Autodesk Fusion 360 part; units mm, degrees
sketch "Sketch1" plane through (0, 0, 0) normal (0, 1, 0) x (1, 0, 0)
  line L0 (35, 20) -> (-35, 20)
  line L1 (-40, 15) -> (-40, -15)
  line L2 (-35, -20) -> (35, -20)
  line L3 (40, -15) -> (40, 15)
  line L4 (40, 20) -> (-40, -20) construction
  line L5 (-40, 20) -> (40, -20) construction
  arc A0 (-35, 20) -> (-40, 15) centre (-35, 15) ccw
  arc A1 (40, 15) -> (35, 20) centre (35, 15) ccw
  arc A2 (35, -20) -> (40, -15) centre (35, -15) ccw
  arc A3 (-40, -15) -> (-35, -20) centre (-35, -15) ccw
  line L6 (-36, 15) -> (-36, -15)
  arc A4 (-36, -15) -> (-35, -16) centre (-35, -15) ccw
  line L7 (-35, -16) -> (35, -16)
  arc A5 (35, -16) -> (36, -15) centre (35, -15) ccw
  line L8 (36, -15) -> (36, 15)
  arc A6 (36, 15) -> (35, 16) centre (35, 15) ccw
  line L9 (35, 16) -> (-35, 16)
  arc A7 (-35, 16) -> (-36, 15) centre (-35, 15) ccw
  dimension "d1" = 80
  dimension "d2" = 40
  dimension "d3" = 5
  dimension "d4" = -4
extrude "Extrude1" add sketch "Sketch1" along normal blind 4 contours L6 A4 L7 A5 L8 A6 L9 A7
extrude "Extrude2" add sketch "Sketch1" along normal blind 20
sketch "Sketch2" plane through (0, 20, 0) normal (0, 1, 0) x (-1, 0, 0)
  arc A0 (35, -16) -> (36, -15) centre (35, -15) ccw
  line L0 (35, -16) -> (-35, -16)
  arc A1 (-36, -15) -> (-35, -16) centre (-35, -15) ccw
  line L1 (-36, -15) -> (-36, 15)
  arc A2 (-35, 16) -> (-36, 15) centre (-35, 15) ccw
  line L2 (-35, 16) -> (35, 16)
  arc A3 (36, 15) -> (35, 16) centre (35, 15) ccw
  line L3 (36, 15) -> (36, -15)
  arc A4 (40, 15) -> (35, 20) centre (35, 15) ccw
  line L4 (35, 20) -> (-35, 20)
  arc A5 (-35, 20) -> (-40, 15) centre (-35, 15) ccw
  line L5 (-40, 15) -> (-40, -15)
  arc A6 (-40, -15) -> (-35, -20) centre (-35, -15) ccw
  line L6 (-35, -20) -> (35, -20)
  arc A7 (35, -20) -> (40, -15) centre (35, -15) ccw
  line L7 (40, -15) -> (40, 15)
  line L8 (37.12, 17.12) -> (-37.12, 17.12)
  line L9 (-37.12, 17.12) -> (-37.12, -17.12)
  line L10 (-37.12, -17.12) -> (37.12, -17.12)
  line L11 (37.12, -17.12) -> (37.12, 17.12)
  line L12 (37.12, 17.12) -> (-37.12, -17.12) construction
  line L13 (-37.12, 17.12) -> (37.12, -17.12) construction
  dimension "d9" = 74.24
  dimension "d10" = 34.24
hole "Hole1" at (37.12, 20, 17.12) at (-37.12, 20, 17.12) at (-37.12, 20, -17.12) at (37.12, 20, -17.12) direction (0, -1, 0) diameter 1.471 depth 11 tip angle 118
Verification items for the finished model (mm, model axes). A direction names the side the tool comes from. Round coordinates to 2 decimals unless told otherwise and drop trailing zeros. Loops run counter-clockwise (first coordinate to the right, second up) from the corner with the lowest first, then second, coordinate; pieces in that order, holes last. Notation, with made-up numbers: (12, 47) - (44, 47) arc R26 ccw to (44, 62) - close; hole circle Ø6 at (6.25, 38). An arc over 180 degrees is marked (long way). Write item = value, one per line.
Q1. Tool access check on faces 5 (the flat face through (0, 10, 20)), 6 (the cylindrical face through (36.9, 14.42, -16.42)). Record the directions out of +Z, -Z, +X, -X, +Y, -Y that give a thin tool (end or side, any length) a straight path to the whole face; none if there is none.
Here are the results:
face_5 = +Z, +X, -X, +Y, -Y
face_6 = +Y
Q2. Sectioned sample at A-A on y = 7.75. Record the boundary of the cut face in (x, z), plus the area to 3 significant figures.
Here are the results:
outline = (-40, -15) arc R5 ccw to (-35, -20) - (35, -20) arc R5 ccw to (40, -15) - (40, 15) arc R5 ccw to (35, 20) - (-35, 20) arc R5 ccw to (-40, 15) - close; hole (-36, -15) arc R1 ccw to (-35, -16) - (35, -16) arc R1 ccw to (36, -15) - (36, 15) arc R1 ccw to (35, 16) - (-35, 16) arc R1 ccw to (-36, 15) - close
area = 875 mm^2
Q3. Sectioned sample at B-B on x = 10. Record the boundary of the cut face in (y, z), plus the area to 3 significant figures.
Here are the results:
outline = (0, -20) - (20, -20) - (20, -16) - (4, -16) - (4, 16) - (20, 16) - (20, 20) - (0, 20) - close
area = 288 mm^2
Q4. Mould release check, pull along Z, two halves, no side actions. Record for faces 1 (the conical face through (-37.012, 8.635, 17.189)), 2 (the flat face through (-1, 4, 0)), 3 (the cylindrical face through (39, 10, 18)), 4 (the cylindrical face through (38, 10, -19)): +Z half, -Z half, draft (parallel to the pull), parting line (faces both ways), or undercut.
Here are the results:
face_1 = undercut
face_2 = undercut
face_3 = +Z half
face_4 = -Z half
Q5. Material ranges on L1, parallel to Z at x = -19.5, y = 13.25; L2, parallel to X at y = 12.75, z = -17.12; L3, parallel to Z at x = 37.12, y = 16, recorded low to high.
Here are the results:
L1 = -20 to -16, 16 to 20
L2 = -39.53 to -37.86, -36.38 to 36.38, 37.86 to 39.53
L3 = -19.53 to -17.86, -16.38 to 16.38, 17.86 to 19.53
Q6. Depth check by flat-ended pin: pin 1 (3 mm diameter, centred on x = -14, z = -3, fed in from +Y); pin 2 (1.2 mm diameter, centred on x = -37.12, z = -17.12, fed in from +Y). Enter the tip coordinate at first touch or a pass-through.
Here are the results:
pin_1 = 4
pin_2 = 8.92
Q7. Sectioned sample at C-C on z = -4. Record the boundary of the cut face in (x, y), plus the area to 3 significant figures.
Here are the results:
outline = (-40, 0) - (40, 0) - (40, 20) - (36, 20) - (36, 4) - (-36, 4) - (-36, 20) - (-40, 20) - close
area = 448 mm^2
